The model under review builds one solid part; all positions refer to its coordinate system, in mm. Face numbers are marked on the shaded views. A direction names the side the tool comes from. Give positions to 0.01 mm unless a question says otherwise; leave off trailing zeros. Order: outer loops, then holes, each group sorted by start corner. A loop starts at its lowest first (then second) coordinate and runs counter-clockwise, first axis right, second up. Notation, with made-up numbers: (1, 62.5) - (57, 62.5) arc R7 ccw to (57, 74.5) - close; hole circle Ø2 at (15.25, -34.75). An arc over 180 degrees is marked (long way). Put each result on its own line as item: value.
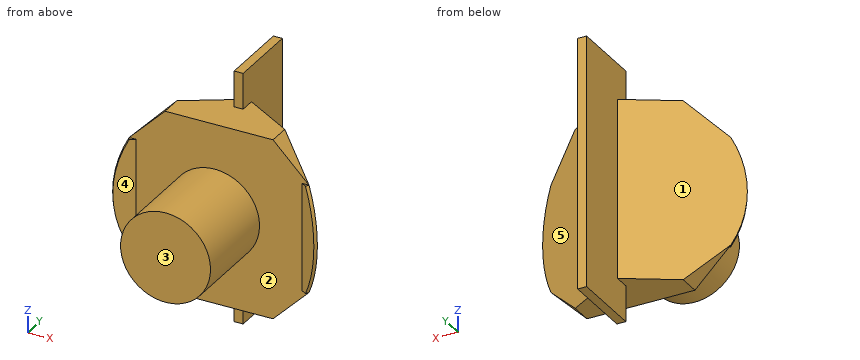
Autodesk Inventor part; units mm, degrees
ref_plane "YZ Plane" through (0, 0, 0) normal (1, 0, 0) x (0, 1, 0)
ref_plane "XZ Plane" through (0, 0, 0) normal (0, 1, 0) x (-1, 0, 0)
ref_plane "XY Plane" through (0, 0, 0) normal (0, 0, 1) x (1, 0, 0)
sketch "Boceto1" plane through (0, 0, 0) normal (0, 0, 1) x (1, 0, 0)
  line L0 (0, 0) -> (-500, 0)
  line L1 (0, 0) -> (500, 0)
  line L2 (0, 0) -> (0, 300)
  line L3 (-500, 0) -> (0, 300)
  line L4 (500, 0) -> (0, 300)
  dimension "d0" = 500
  dimension "d1" = 500
  dimension "d2" = 300
extrude "Extrusión1" add sketch "Boceto1" along normal blind 1000
sketch "Boceto2" plane through (-500, 0, 0) normal (0, -1, 0) x (1, 0, 0)
  line L0 (0, 1000) -> (1000, 1000)
  line L1 (0, 1000) -> (0, 800)
  line L2 (0, 0) -> (0, 1000)
  line L3 (0, 800) -> (200, 1000)
  line L4 (200, 1000) -> (0, 1000)
  line L5 (1000, 1000) -> (800, 1000)
  line L6 (800, 1000) -> (1000, 800)
  line L7 (1000, 0) -> (1000, 1000)
  line L8 (1000, 800) -> (1000, 1000)
  line L9 (0, 0) -> (1000, 0)
  line L10 (0, 0) -> (0, 200)
  line L11 (200, 0) -> (0, 0)
  line L12 (200, 0) -> (0, 200)
  line L13 (1000, 0) -> (800, 0)
  line L14 (800, 0) -> (1000, 0)
  line L15 (1000, 200) -> (800, 0)
  point P0 (500, 0)
  dimension "d5" = 200
  dimension "d6" = 45
  dimension "d7" = 200
  dimension "d8" = 45
extrude "Extrusión2" cut sketch "Boceto2" against normal blind 1000 contours L0 L3 L1 | L0 L7 L6 | L12 L9 L2 | L7 L9 L15
sketch "Boceto3" plane through (0, 300, 1000) normal (0.5145, 0.8575, 0) x (0.8575, -0.5145, 0)
  line L0 (583.0952, 800) -> (583.0952, 200)
  arc A0 (583.0952, 200) -> (583.0952, 800) centre (63.4799, 500) ccw
  line L1 (583.0952, 800) -> (473.0952, 800)
  line L2 (473.0952, 800) -> (473.0952, 200)
  line L3 (473.0952, 200) -> (583.0952, 200)
  line L4 (583.0952, 200) -> (583.0952, 800)
  point P0 (154.3487, 1000)
  dimension "d11" = 600
  dimension "d12" = 110
extrude "Extrusión3" add sketch "Boceto3" against normal blind 20
sketch "Boceto4" plane through (0, 300, 1000) normal (-0.5145, 0.8575, 0) x (0.8575, 0.5145, 0)
  line L0 (-583.0952, 800) -> (-583.0952, 200)
  arc A0 (-583.0952, 800) -> (-583.0952, 200) centre (-63.4799, 500) ccw
  line L1 (-583.0952, 800) -> (-473.0952, 800)
  line L2 (-473.0952, 800) -> (-473.0952, 200)
  line L3 (-473.0952, 200) -> (-583.0952, 200)
  line L4 (-583.0952, 200) -> (-583.0952, 800)
  point P0 (-154.3487, 1000)
  dimension "d15" = 600
  dimension "d16" = 110
extrude "Extrusión4" add sketch "Boceto4" against normal blind 20
sketch "Boceto5" plane through (0, 0, 0) normal (0, 0, -1) x (-1, 0, 0)
  line L0 (-300, 120) -> (0, 300)
  line L1 (0, 300) -> (0, 200)
  line L2 (0, 200) -> (25, 200)
  line L3 (0, 200) -> (-25, 200)
  line L4 (-25, 200) -> (-25, 600)
  line L5 (-25, 600) -> (25, 600)
  line L6 (25, 600) -> (25, 200)
  point P0 (0, 0)
  dimension "d19" = 100
  dimension "d20" = 25
  dimension "d21" = 25
  dimension "d22" = 400
extrude "Extrusión5" add sketch "Boceto5" along normal blind 200 and the other way blind 1200
sketch "Boceto6" plane through (-300, 0, 0) normal (0, -1, 0) x (1, 0, 0)
  line L0 (275, 1000) -> (275, 0)
  circle A0 centre (275, 500) radius 250
  point P0 (300, 0)
  dimension "d27" = 500
extrude "Extrusión6" add sketch "Boceto6" along normal blind 500
properties part number "Base_rotativa"
(1) For the marked faces 1 and 2, list the 3-axis set-ups (+Z, -Z, +X, -X, +Y, -Y) from which the entire face can be reached by the end or side of a thin tool; tool diameter is ignored.
The answers:
face 1: +Z, -Z, -X, +Y
face 2: -Y
(2) Clearance check with flat-ended pins moving along their axes: pin 1 Ø3 at (y, z) = (199.5, 972) entering from +X; pin 2 Ø8.5 at (x, y) = (479, -5.5) entering from +Z; pin 3 Ø15 at (x, z) = (0.5, 1058) entering from -Y. State where each tip first meets the part, or that it passes through.
The answers:
pin 1: x = 170
pin 2: z = 800
pin 3: y = 200
(3) Take a section at B-B, the plane z = 500. Write out the cut boundary in (x, y).
The answers:
outline: (-568.93, -41.36) - (-558.64, -58.51) - (-461.13, 0) - (-275, 0) - (-275, -500) - (225, -500) - (225, 0) - (461.13, 0) - (558.64, -58.51) - (568.93, -41.36) - (25, 285) - (25, 600) - (-25, 600) - (-25, 285) - close
(4) Take a section at A-A, the plane y = 87. Write out the cut boundary in (x, z), then the cut area to 3 significant figures.
The answers:
outline: (-355, 55) - (-300, 0) - (300, 0) - (355, 55) - (355, 945) - (300, 1000) - (-300, 1000) - (-355, 945) - close
area: 704,000 mm^2
(5) Take a section at D-D, the plane y = -392. Write out the cut boundary in (x, z).
The answers:
outline: circle Ø500 at (-25, 500)
(6) Take a section at C-C, the plane x = -332. Write out the cut boundary in (y, z).
The answers:
outline: (0, 32) - (100.8, 32) - (100.8, 968) - (0, 968) - close
(7) Wall thickness on L1, parallel to X at y = -19.5, z = 321; L2, parallel to X at y = 261, z = -46.5; L3, parallel to Z at x = 39.5, y = 101.5: over which ranges is each line inside the solid? List them lowest first.
The answers:
L1: -532.5 to -493.63, -199.53 to 149.53, 493.63 to 532.5
L2: -25 to 25
L3: 0 to 1000
(8) The part is to be moulded in two halves that separate along X. For the marked faces 3, 4 and 5, say which applies: pulls with the +X half, pulls with the -X half, needs draft (parallel to the pull), parting line crosses it, or undercut.
The answers:
face 3: needs draft
face 4: undercut
face 5: pulls with the +X half
